Could you check a few things on this model? Use its own coordinates, in mm. Face numbers are marked on the shaded views. A direction names the side the tool comes from. Give positions to 0.01 mm unless a question says otherwise; leave off trailing zeros. Loops run counter-clockwise (first coordinate to the right, second up) from the corner with the lowest first, then second, coordinate; pieces in that order, holes last. Notation, with made-up numbers: M -12,17 L 23,17 A23 cw 23,33 Z; hole C 46,43.25 d11. An arc over 180 degrees is marked long. Answer in a Markdown table with one row per item. Add a question column.
1. If we section it at B-B on y = 0: List the corners of the cut face in (x, z) for me.
2. If we section it at C-C on x = 37.5: List the corners of the cut face in (y, z) for me, then the cut area to 3 significant figures.
3. I need wall thicknesses on line 1 along X through (y, z) = (-5.25, 0); line 2 along X through (y, z) = (-2.25, -4); line 3 along X through (y, z) = (1, 0). Which ranges of each line are inside material? Lowest first, please. Write a range as from..to.
4. If we section it at A-A on z = 0: List the corners of the cut face in (x, y) for me.
5. I'm going to push flat-ended pins straight in: pin 1 Ø2 at (x, y) = (-18.5, -5.5) entering from +Z; pin 2 Ø10 at (x, y) = (-32.5, 8) entering from +Z; pin 3 Ø12 at (x, z) = (24, 8.5) entering from +Y. Where does each tip first touch, or does it pass through?
6. If we section it at D-D on x = 63: List the corners of the cut face in (y, z) for me, then the cut area to 3 significant figures.
7. Which directions (+Z, -Z, +X, -X, +Y, -Y) give clear straight access to the entire face, cutting with the end or side of a thin tool? Please do the marked faces 1, 2 and 3.
```python
from build123d import *

# Parameters (mm, degrees)
CUT_EXTRUDE1_DEPTH      = 79.774764709
CUT_EXTRUDE1_DEPTH_BACK = 79.774764709
SKETCH2_R               = 3


with BuildPart() as part:
    # Sketch1 → Revolve1 (revolve)
    with BuildSketch(Plane.XY):
        Polygon((41, 4.267874105), (51, 4.267874105), (51, 10.774632754), (75, 10.774632754), (75, 0), (-63, 0), (-63, 6), (-56, 6), (-56, 4), (-50, 4), (-50, 6), (-41, 6), (-41, 8), (41, 8), align=None)
    revolve(axis=Axis((75, 0, 0), (-1, 0, 0)))

    # Sketch2 → Cut-Extrude1 (cut, two sides: drawn at the far end of the back side and taken through both)
    with BuildSketch(Plane(origin=(0, 10.774632754, 0), x_dir=(1, 0, 0), z_dir=(0, 1, 0)).offset(-CUT_EXTRUDE1_DEPTH_BACK)):
        with Locations(Location((63, 0, 0), (0, 0, 180))):
            Circle(SKETCH2_R)
    extrude(amount=CUT_EXTRUDE1_DEPTH + CUT_EXTRUDE1_DEPTH_BACK, mode=Mode.SUBTRACT)


solid = part.part
```
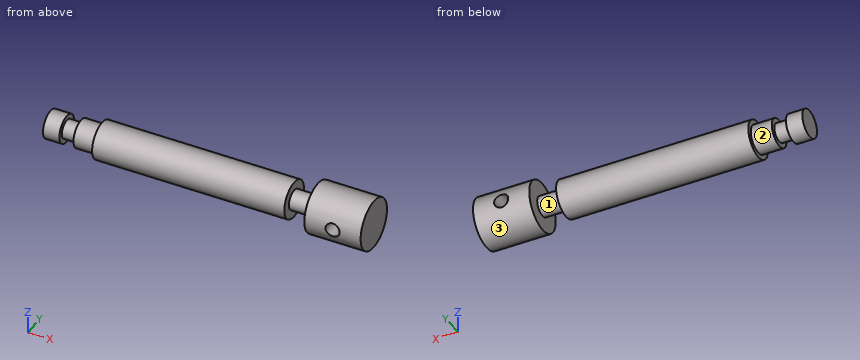
Results:
| question | item | result |
|---|---|---|
| 1 | outline | M -63,-6 L -56,-6 L -56,-4 L -50,-4 L -50,-6 L -41,-6 L -41,-8 L 41,-8 L 41,-4.27 L 51,-4.27 L 51,-10.77 L 75,-10.77 L 75,10.77 L 51,10.77 L 51,4.27 L 41,4.27 L 41,8 L -41,8 L -41,6 L -50,6 L -50,4 L -56,4 L -56,6 L -63,6 Z; hole C 63,0 d6 |
| 2 | outline | C 0,0 d16 |
| 2 | area | 201 mm2 |
| 3 | line 1 | -63..-56, -50..41, 51..60, 66..75 |
| 3 | line 2 | -63..-56, -50..41, 51..75 |
| 3 | line 3 | -63..60, 66..75 |
| 4 | outline | M -63,-6 L -56,-6 L -56,-4 L -50,-4 L -50,-6 L -41,-6 L -41,-8 L 41,-8 L 41,-4.27 L 51,-4.27 L 51,-10.77 L 60,-10.77 L 60,10.77 L 51,10.77 L 51,4.27 L 41,4.27 L 41,8 L -41,8 L -41,6 L -50,6 L -50,4 L -56,4 L -56,6 L -63,6 Z; M 66,-10.77 L 75,-10.77 L 75,10.77 L 66,10.77 Z |
| 5 | pin 1 | z = 6.61 |
| 5 | pin 2 | z = 7.42 |
| 5 | pin 3 | y = 7.6 |
| 6 | outline | M -10.35,-3 A10.77 ccw 10.35,-3 Z; M -10.35,3 L 10.35,3 A10.77 ccw Z |
| 6 | area | 237 mm2 |
| 7 | face 1 | none |
| 7 | face 2 | -X |
| 7 | face 3 | +X, -X |
